Build history of the part. All positions in model axes, mm. A direction names the side the tool comes from. Coordinates: 2 decimals unless noted, no trailing zeros. Order: outer loops, then holes, each group sorted by start corner. A loop starts at its lowest first (then second) coordinate and runs counter-clockwise, first axis right, second up. Notation, with made-up numbers: (69.25, 55) - (95.25, 55) arc R22 cw to (95.25, 63) - close; hole circle Ø2 at (28, 44.5). An arc over 180 degrees is marked (long way). Write each question's results on one line, items separated by ' | '.
from build123d import *

# Parameters (mm, degrees)
CROQUIS1_W               = 154
CROQUIS1_H               = 71
SALIENTE_EXTRUIR1_DEPTH  = 1.5
CROQUIS2_W               = 12
CROQUIS2_H               = 3
CROQUIS2_W_2             = 10
CROQUIS2_W_3             = 3
CROQUIS2_H_2             = 11
CROQUIS2_H_3             = 5
CORTAR_EXTRUIR1_DEPTH    = 13
CROQUIS4_W               = 30
CROQUIS4_H               = 3
SALIENTE_EXTRUIR3_DEPTH  = 3
REDONDEO2_R              = 3
CROQUIS5_R               = 1.5
CORTAR_EXTRUIR2_DEPTH    = 3
REDONDEO2_OF_SIMETR_A4_R = 3
SIMETR_A5_START          = -2
SIMETR_A5_OUTLINE_R      = 1.5
SIMETR_A5_DEPTH          = 4
SIMETR_A5_START_2        = -1.5
SIMETR_A5_2_DEPTH        = 3
CROQUIS6_W               = 3
CROQUIS6_H               = 10
CROQUIS6_W_2             = 9.7
CROQUIS6_H_2             = 2.94
CROQUIS6_W_3             = 10.628979849
CROQUIS6_H_3             = 19.526562675
CORTAR_EXTRUIR3_DEPTH    = 10
CROQUIS7_R               = 1.5
CORTAR_EXTRUIR4_DEPTH    = 10
CROQUIS8_W               = 9
CROQUIS8_H               = 3
CORTAR_EXTRUIR5_DEPTH    = 10
CROQUIS9_R               = 1.3
CORTAR_EXTRUIR6_DEPTH    = 10
CROQUIS10_W              = 2.94
CROQUIS10_H              = 4.8
CORTAR_EXTRUIR7_DEPTH    = 23


with BuildPart() as part:
    # Croquis1 → Saliente-Extruir1 (new, symmetric)
    with BuildSketch(Plane(origin=(0, 0, 0), x_dir=(0, 0, -1), z_dir=(1, 0, 0))):
        Rectangle(CROQUIS1_W, CROQUIS1_H)
    extrude(amount=SALIENTE_EXTRUIR1_DEPTH, both=True)

    # Croquis2 → Cortar-Extruir1 (cut)
    with BuildSketch(Plane(origin=(1.5, 0, 0), x_dir=(0, 0, -1), z_dir=(1, 0, 0))):
        with Locations((-71, 34)):
            Rectangle(CROQUIS2_W, CROQUIS2_H)
        with Locations((-50, 34)):
            Rectangle(CROQUIS2_W_2, CROQUIS2_H)
        with Locations((-10, 34)):
            Rectangle(CROQUIS2_W_2, CROQUIS2_H)
        with Locations((10, 34)):
            Rectangle(CROQUIS2_W_2, CROQUIS2_H)
        with Locations((50, 34)):
            Rectangle(CROQUIS2_W_2, CROQUIS2_H)
        with Locations((71, 34)):
            Rectangle(CROQUIS2_W, CROQUIS2_H)
        with Locations((50, -34)):
            Rectangle(CROQUIS2_W_2, CROQUIS2_H)
        with Locations((10, -34)):
            Rectangle(CROQUIS2_W_2, CROQUIS2_H)
        with Locations((-10, -34)):
            Rectangle(CROQUIS2_W_2, CROQUIS2_H)
        with Locations((-50, -34)):
            Rectangle(CROQUIS2_W_2, CROQUIS2_H)
        with Locations((-71, -34)):
            Rectangle(CROQUIS2_W, CROQUIS2_H)
        with Locations((71, -34)):
            Rectangle(CROQUIS2_W, CROQUIS2_H)
        with Locations((-75.5, -16)):
            Rectangle(CROQUIS2_W_3, CROQUIS2_H_2)
        with Locations((-75.5, 0)):
            Rectangle(CROQUIS2_W_3, CROQUIS2_H_3)
        with Locations((-75.5, 16)):
            Rectangle(CROQUIS2_W_3, CROQUIS2_H_2)
        with Locations((75.5, -16)):
            Rectangle(CROQUIS2_W_3, CROQUIS2_H_2)
        with Locations((75.5, 16)):
            Rectangle(CROQUIS2_W_3, CROQUIS2_H_2)
        with Locations((75.5, 0)):
            Rectangle(CROQUIS2_W_3, CROQUIS2_H_3)
    extrude(amount=-CORTAR_EXTRUIR1_DEPTH, mode=Mode.SUBTRACT)

    # Croquis4 → Saliente-Extruir3 (add)
    with BuildSketch(Plane(origin=(1.5, 0, 0), x_dir=(0, 0, -1), z_dir=(1, 0, 0))):
        with Locations((-30, 37)):
            Rectangle(CROQUIS4_W, CROQUIS4_H)
    saliente_extruir3 = extrude(amount=-SALIENTE_EXTRUIR3_DEPTH)

    # Redondeo2
    redondeo2_edges = [part.edges().sort_by_distance(p)[0] for p in [
        (0, 38.5, 45),
        (0, 38.5, 15),
    ]]
    fillet(redondeo2_edges, radius=REDONDEO2_R)

    # Croquis5 → Cortar-Extruir2 (cut)
    with BuildSketch(Plane(origin=(1.5, 0, 0), x_dir=(0, 0, -1), z_dir=(1, 0, 0))):
        with Locations((-30, 34)):
            Circle(CROQUIS5_R)
    cortar_extruir2 = extrude(amount=-CORTAR_EXTRUIR2_DEPTH, mode=Mode.SUBTRACT)

    # Simetría4: Saliente-Extruir3, Cortar-Extruir2 across plane
    add(saliente_extruir3.mirror(Plane.ZX))
    add(cortar_extruir2.mirror(Plane.ZX), mode=Mode.SUBTRACT)

    # Redondeo2 of Simetría4
    redondeo2_of_simetr_a4_edges = [part.edges().sort_by_distance(p)[0] for p in [
        (0, -38.5, 45),
        (0, -38.5, 15),
    ]]
    fillet(redondeo2_of_simetr_a4_edges, radius=REDONDEO2_OF_SIMETR_A4_R)

    # Simetría5: read off the stored shape, not the designer's step
    # Simetría5 outline → Simetría5 (cut)
    with BuildSketch(Plane.YZ.offset(SIMETR_A5_START)):
        with Locations((34, -30)):
            Circle(SIMETR_A5_OUTLINE_R)
        with Locations((-34, -30)):
            Circle(SIMETR_A5_OUTLINE_R)
    extrude(amount=SIMETR_A5_DEPTH, mode=Mode.SUBTRACT)

    # Simetr_a5 2 outline → Simetr_a5 2 (add)
    with BuildSketch(Plane.YZ.offset(SIMETR_A5_START_2)):
        with BuildLine():
            Line((38.5, -42), (38.5, -18))
            ThreePointArc((38.5, -18), (37.621320344, -15.878679656), (35.5, -15))
            Line((35.5, -15), (35.5, -45))
            ThreePointArc((35.5, -45), (37.621320344, -44.121320344), (38.5, -42))
        make_face()
        with BuildLine():
            ThreePointArc((-35.5, -15), (-37.621320344, -15.878679656), (-38.5, -18))
            Line((-38.5, -18), (-38.5, -42))
            ThreePointArc((-38.5, -42), (-37.621320344, -44.121320344), (-35.5, -45))
            Line((-35.5, -45), (-35.5, -15))
        make_face()
    extrude(amount=SIMETR_A5_2_DEPTH)

    # Croquis6 → Cortar-Extruir3 (cut)
    with BuildSketch(Plane.ZY.offset(1.5)):
        with Locations((47.6, -15.1)):
            Rectangle(CROQUIS6_W, CROQUIS6_H)
        with Locations((47.6, 19.9)):
            Rectangle(CROQUIS6_W, CROQUIS6_H)
        with Locations((-47.6, -15.1)):
            Rectangle(CROQUIS6_W, CROQUIS6_H)
        with Locations((-47.6, 19.9)):
            Rectangle(CROQUIS6_W, CROQUIS6_H)
        with Locations((15, -27)):
            Rectangle(CROQUIS6_W_2, CROQUIS6_H_2)
        with Locations((64, -27)):
            Rectangle(CROQUIS6_W_2, CROQUIS6_H_2)
        with Locations((-64, -27)):
            Rectangle(CROQUIS6_W_2, CROQUIS6_H_2)
        with Locations((-15, -27)):
            Rectangle(CROQUIS6_W_2, CROQUIS6_H_2)
        with Locations((0.209178282, -13.227366202)):
            Rectangle(CROQUIS6_W_3, CROQUIS6_H_3)
    extrude(amount=-CORTAR_EXTRUIR3_DEPTH, mode=Mode.SUBTRACT)

    # Croquis7 → Cortar-Extruir4 (cut)
    with BuildSketch(Plane(origin=(1.5, 0, 0), x_dir=(0, 0, -1), z_dir=(1, 0, 0))):
        with Locations((-47.6, -4.7)):
            Circle(CROQUIS7_R)
        with Locations(Location((47.6, -4.7, 0), (0, 0, 180))):
            Circle(CROQUIS7_R)
    extrude(amount=-CORTAR_EXTRUIR4_DEPTH, mode=Mode.SUBTRACT)

    # Croquis8 → Cortar-Extruir5 (cut)
    with BuildSketch(Plane.ZY.offset(1.5)):
        with Locations((-33.6, -11)):
            Rectangle(CROQUIS8_W, CROQUIS8_H)
        with Locations((-61.6, -11)):
            Rectangle(CROQUIS8_W, CROQUIS8_H)
        with Locations((33.6, -11)):
            Rectangle(CROQUIS8_W, CROQUIS8_H)
        with Locations((61.6, -11)):
            Rectangle(CROQUIS8_W, CROQUIS8_H)
    extrude(amount=-CORTAR_EXTRUIR5_DEPTH, mode=Mode.SUBTRACT)

    # Croquis9 → Cortar-Extruir6 (cut)
    with BuildSketch(Plane(origin=(1.5, 0, 0), x_dir=(0, 0, -1), z_dir=(1, 0, 0))):
        with Locations((-23, 0)):
            Circle(CROQUIS9_R)
        with Locations((7, 10.5)):
            Circle(CROQUIS9_R)
        with Locations((7, -10.5)):
            Circle(CROQUIS9_R)
    extrude(amount=-CORTAR_EXTRUIR6_DEPTH, mode=Mode.SUBTRACT)

    # Croquis10 → Cortar-Extruir7 (cut)
    with BuildSketch(Plane.ZY.offset(1.5)):
        with Locations((-19.8, 12.5)):
            Rectangle(CROQUIS10_W, CROQUIS10_H)
        with Locations((-19.8, -13)):
            Rectangle(CROQUIS10_W, CROQUIS10_H)
        with Locations((19.8, 12.5)):
            Rectangle(CROQUIS10_W, CROQUIS10_H)
        with Locations((19.8, -13)):
            Rectangle(CROQUIS10_W, CROQUIS10_H)
    extrude(amount=-CORTAR_EXTRUIR7_DEPTH, mode=Mode.SUBTRACT)


solid = part.part
1. Drop flat-ended pins along their axis: pin 1 Ø0.9 at (x, z) = (-0.5, -48.5) entering from -Y; pin 2 Ø2.5 at (y, z) = (-34, -30) entering from -X; pin 3 Ø1.5 at (x, y) = (0.5, -14) entering from -Z; pin 4 Ø1 at (x, z) = (-1, 61) entering from -Y. Give the stop position or say it passes through.
Solved:
pin 1: stops at y = -32.5 | pin 2: passes through | pin 3: stops at z = -74 | pin 4: stops at y = -35.5
2. Two-plate mould, pull along Y, no slides. Class faces 5 (the face through (0, -32.5, -10)), 6 (the face through (0, -11, 38.1)), 7 (the face through (0, 32.5, 10)), 8 (the face through (0, -25.53, -64)): +Y half, -Y half, draft (parallel to the pull), parting line (faces both ways), or undercut.
Solved:
face 5: -Y half | face 6: undercut | face 7: +Y half | face 8: undercut
3. Band-saw the part on D-D on x = -0.5. Give the number of separate pieces and of enclosed holes in the cut face, then the cut area to 3 significant figures.
Solved:
separate pieces: 1 | enclosed holes: 26 | area: 10,100 mm2
4. Tool access for faces 1 (the face through (0, -16, -74)), 2 (the face through (0, 34, -65)), 3 (the face through (0, 2.5, 76)), 4 (the face through (0, -12.5, 34)): list every direction of +Z, -Z, +X, -X, +Y, -Y with a clear straight run to the whole face (end or side of a thin tool).
Solved:
face 1: -Z, +X, -X | face 2: -Z, +X, -X, +Y | face 3: +Z, +X, -X | face 4: +X, -X
5. Probe line 1 (Y direction, x = -0.2, z = -47.6); line 2 (Y direction, x = 0.75, z = -7); line 3 (Z direction, x = -0.35, y = -19). List the from-to ranges inside material, lowest first.
Solved:
line 1: y = -32.5 to -20.1, -10.1 to -6.2, -3.2 to 14.9, 24.9 to 32.5 | line 2: y = -32.5 to -11.8, -9.2 to 9.2, 11.8 to 32.5 | line 3: z = -74 to -49.1, -46.1 to -5.11, 5.52 to 46.1, 49.1 to 74
6. Band-saw the part on C-C on y = 34. Give the cut face in (x, z), then the cut area to 3 significant figures.
Solved:
outline: (-1.5, -65) - (1.5, -65) - (1.5, -55) - (-1.5, -55) - close; (-1.5, -45) - (1.5, -45) - (1.5, -31.5) - (-1.5, -31.5) - close; (-1.5, -28.5) - (1.5, -28.5) - (1.5, -15) - (-1.5, -15) - close; (-1.5, -5) - (1.5, -5) - (1.5, 5) - (-1.5, 5) - close; (-1.5, 15) - (1.5, 15) - (1.5, 28.5) - (-1.5, 28.5) - close; (-1.5, 31.5) - (1.5, 31.5) - (1.5, 45) - (-1.5, 45) - close; (-1.5, 55) - (1.5, 55) - (1.5, 65) - (-1.5, 65) - close | area: 252 mm2
7. Band-saw the part on B-B on y = 17. Give the cut face in (x, z).
Solved:
outline: (-1.5, -74) - (1.5, -74) - (1.5, -49.1) - (-1.5, -49.1) - close; (-1.5, -46.1) - (1.5, -46.1) - (1.5, 46.1) - (-1.5, 46.1) - close; (-1.5, 49.1) - (1.5, 49.1) - (1.5, 74) - (-1.5, 74) - close
8. Band-saw the part on A-A on z = 47.6. Give the cut face in (x, y).
Solved:
outline: (-1.5, -32.5) - (1.5, -32.5) - (1.5, -20.1) - (-1.5, -20.1) - close; (-1.5, -10.1) - (1.5, -10.1) - (1.5, -6.2) - (-1.5, -6.2) - close; (-1.5, -3.2) - (1.5, -3.2) - (1.5, 14.9) - (-1.5, 14.9) - close; (-1.5, 24.9) - (1.5, 24.9) - (1.5, 32.5) - (-1.5, 32.5) - close
